Geometry check sheet. Reference: the model listing, model coordinates, mm. A direction names the side the tool comes from. Give positions to 0.01 mm unless a question says otherwise; leave off trailing zeros. Write each loop counter-clockwise with the first axis right and the second up, starting at its lowest first coordinate (ties: lowest second). Pieces come first, ordered by that corner, then holes. Notation, with made-up numbers: (60, 38) - (114, 38) arc R31 cw to (114, 71) - close; hole circle Ø6 at (-12, -17). An arc over 180 degrees is marked (long way). Write item = value, one per line. Start each with the question number.
(1) Section check A-A, the plane x = 0. Enter the section's corners in (y, z), plus the area to 3 significant figures.
(2) Depth check by flat-ended pin: pin 1 Ø12.5 at (x, y) = (5, 0.5) entering from +Z; pin 2 Ø10 at (x, z) = (-17.5, 17.5) entering from +Y; pin 3 Ø1.5 at (x, z) = (31, 84.5) entering from -Y. Enter the tip coordinate at first touch or a pass-through.
(3) Draft check along X on faces 3 (the cylindrical face through (11.923, 3.755, 75.35)), 4 (the flat face through (0, 0, 50)), 5 (the flat face through (6, 77, 0)), 6 (the cylindrical face through (-60.742, 69.964, -4.93)). Enter one of: pulls with the +X half, pulls with the -X half, needs draft (parallel to the pull), parting line crosses it, or undercut.
(4) Access from +Z, -Z, +X, -X, +Y, -Y to the whole of each face (thin tool, end or side, straight path). Record for faces 1 (the flat face through (75, 0, -5)), 2 (the flat face through (6, -77, 0)).
(5) Section check B-B, the plane z = 59.5. Enter the section's corners in (x, y).
(6) Section check C-C, the plane z = 31. Enter the section's corners in (x, y).
(7) Thickness scan on L1, parallel to Z at x = 53.5, y = 55; L2, parallel to Y at x = 0, z = 77; L3, parallel to Y at x = -0.5, z = 71. Record the ranges inside material, lowest first.
```python
from build123d import *

# Parameters (mm, degrees)
SKETCH1_R           = 75
BOSS_EXTRUDE1_DEPTH = 100
BOSS_EXTRUDE1_TAPER = 3
BOSS_EXTRUDE2_DEPTH = 10
SKETCH3_R           = 12.5
CUT_EXTRUDE1_DEPTH  = 50


with BuildPart() as part:
    # Sketch1 → Boss-Extrude1 (new body)
    with BuildSketch(Plane.XY):
        Circle(SKETCH1_R)
    extrude(amount=BOSS_EXTRUDE1_DEPTH, taper=BOSS_EXTRUDE1_TAPER)

    # Sketch2 → Boss-Extrude2 (add)
    with BuildSketch(Plane(origin=(0, 0, 0), x_dir=(-1, 0, 0), z_dir=(0, 0, -1))):
        with BuildLine():
            Line((-25, -85), (25, -85))
            ThreePointArc((25, -85), (60.355339059, -70.355339059), (75, -35))
            Line((75, -35), (75, 35))
            ThreePointArc((75, 35), (60.355339059, 70.355339059), (25, 85))
            Line((25, 85), (-25, 85))
            ThreePointArc((-25, 85), (-60.355339059, 70.355339059), (-75, 35))
            Line((-75, 35), (-75, -35))
            ThreePointArc((-75, -35), (-60.355339059, -70.355339059), (-25, -85))
        make_face()
    extrude(amount=BOSS_EXTRUDE2_DEPTH)

    # Sketch3 → Cut-Extrude1 (cut)
    with BuildSketch(Plane.XY.offset(100)):
        Circle(SKETCH3_R)
    extrude(amount=-CUT_EXTRUDE1_DEPTH, mode=Mode.SUBTRACT)


solid = part.part
```
Model answer:
q1.outline = (-85, -10) - (85, -10) - (85, 0) - (75, 0) - (69.76, 100) - (12.5, 100) - (12.5, 50) - (-12.5, 50) - (-12.5, 100) - (-69.76, 100) - (-75, 0) - (-85, 0) - close
q1.area = 14,900 mm²
q2.pin_1 = 50
q2.pin_2 = 73.06
q2.pin_3 = -63.76
q3.face_3 = undercut
q3.face_4 = undercut
q3.face_5 = needs draft
q3.face_6 = pulls with the -X half
q4.face_1 = +Z, -Z, +X, +Y, -Y
q4.face_2 = +Z, -Y
q5.outline = circle Ø143.76 at (0, 0); hole circle Ø25 at (0, 0)
q6.outline = circle Ø146.75 at (0, 0)
q7.L1 = -10 to 0
q7.L2 = -70.96 to -12.5, 12.5 to 70.96
q7.L3 = -71.28 to -12.49, 12.49 to 71.28
